```python
from build123d import *

# Parameters (mm, degrees)
F1_DEPTH    = 12.4968
F3_DEPTH    = 152.4
F4_T1_DEPTH = 61.7762374031
F5_R        = 5.08


# Not quite as in the source:
# - a fillet or chamfer that OpenCascade refuses, or shapes differently, is made with other operations: its cross-section is extruded or revolved along the edge and cut away or added
# - a feature names something its author has since deleted; it is built from what else it names


with BuildPart() as f1:
    # F0 (on Top) → F1 (new body)
    with BuildSketch(Plane.XY):
        with BuildLine():
            Line((-93.9849921167, 7.4851757918), (-16.1919427612, 7.4851757918))
            ThreePointArc((-16.1919427612, 7.4851757918), (-15.8959532901, 11.2229099464), (-15.7736930996, 14.9703515835))
            Line((-15.7736930996, 14.9703515835), (-93.9849921167, 14.9703515835))
            Line((-93.9849921167, 14.9703515835), (-93.9849921167, 7.4851757918))
        make_face()
        with BuildLine():
            Line((-93.9849921167, 0), (-17.3162451786, 0))
            ThreePointArc((-17.3162451786, 0), (-16.6663908007, 3.7294145399), (-16.1919427612, 7.4851757918))
            Line((-16.1919427612, 7.4851757918), (-93.9849921167, 7.4851757918))
            Line((-93.9849921167, 7.4851757918), (-93.9849921167, 0))
        make_face()
        Polygon((-93.9849921167, -14.5700745956), (-93.9849921167, 0), (-93.9849921167, 7.4851757918), (-93.9849921167, 14.9703515835), (-93.9849921167, 40.6753872946), (-111.9173921167, 19.2205523892), (-111.9173921167, 14.5700745956), (-111.9173921167, -14.5700745956), align=None)
        with BuildLine():
            Line((-15.7736930996, 14.9703515835), (-8.9203921167, 14.9703515835))
            ThreePointArc((-8.9203921167, 14.9703515835), (-14.3796310702, 36.1097695722), (-23.5038306564, 55.9447705746))
            Line((-23.5038306564, 55.9447705746), (-36.6789735854, 66.7365342379))
            Line((-36.6789735854, 66.7365342379), (-31.7310467362, 54.1373938322))
            ThreePointArc((-31.7310467362, 54.1373938322), (-21.3821676169, 35.5195355237), (-15.7736930996, 14.9703515835))
        make_face()
        with BuildLine():
            Line((-17.3162451786, 0), (-8.9203921167, 0))
            ThreePointArc((-8.9203921167, 0), (-8.270322019, 3.7175238692), (-8.0526666958, 7.4851757917))
            Line((-8.0526666958, 7.4851757918), (-16.1919427612, 7.4851757918))
            ThreePointArc((-16.1919427612, 7.4851757918), (-16.6663908007, 3.7294145399), (-17.3162451786, 0))
        make_face()
        with BuildLine():
            Line((-16.1919427612, 7.4851757918), (-8.0526666958, 7.4851757918))
            ThreePointArc((-8.0526666958, 7.4851757917), (-8.270322019, 11.2528277143), (-8.9203921167, 14.9703515835))
            Line((-8.9203921167, 14.9703515835), (-15.7736930996, 14.9703515835))
            ThreePointArc((-15.7736930996, 14.9703515835), (-15.8959532901, 11.2229099464), (-16.1919427612, 7.4851757918))
        make_face()
        with BuildLine():
            ThreePointArc((-34.6760861576, -35.9113998711), (-16.812117143, -21.5317519133), (-8.9203921167, 0))
            Line((-8.9203921167, 0), (-17.3162451786, 0))
            ThreePointArc((-17.3162451786, 0), (-24.4639001208, -18.231884723), (-37.7452522516, -32.6227247715))
            Line((-37.7452522516, -32.6227247715), (-41.4012260735, -32.6227247715))
            Line((-41.4012260735, -32.6227247715), (-41.4012260735, -41.2478148937))
            Line((-41.4012260735, -41.2478148937), (-39.2100475191, -41.5528100016))
            Line((-39.2100475191, -41.5528100016), (-39.2100475191, -49.5910942554))
            Line((-39.2100475191, -49.5910942554), (-34.6760861576, -49.5910942554))
            Line((-34.6760861576, -49.5910942554), (-34.6760861576, -35.9113998711))
        make_face()
        with BuildLine():
            ThreePointArc((-8.9203921167, 14.9703515835), (-8.270322019, 11.2528277143), (-8.0526666958, 7.4851757917))
            Line((-8.0526666958, 7.4851757918), (16.7025048286, 7.4851757918))
            Line((16.7025048286, 7.4851757918), (16.7025048286, 14.9703515835))
            Line((16.7025048286, 14.9703515835), (-8.9203921167, 14.9703515835))
        make_face()
        with BuildLine():
            ThreePointArc((-8.0526666958, 7.4851757917), (-8.270322019, 3.7175238692), (-8.9203921167, 0))
            Line((-8.9203921167, 0), (16.7025048286, 0))
            Line((16.7025048286, 0), (16.7025048286, 7.4851757918))
            Line((16.7025048286, 7.4851757918), (-8.0526666958, 7.4851757918))
        make_face()
        Polygon((16.7025048286, 7.4851757918), (16.7025048286, 0), (33.5264503956, 7.4851757918), (16.7025048286, 14.9703515835), align=None)
    extrude(amount=F1_DEPTH)

    # F2 (on face) → F3 (cut)
    with BuildSketch(Plane(origin=(-111.9173921167, 0, 0), x_dir=(0, -1, 0), z_dir=(-1, 0, 0))):
        with BuildLine():
            ThreePointArc((-5.9230757918, 6.2484), (-6.3806042889, 7.3529715029), (-7.4851757918, 7.8105))
            Line((-7.4851757918, 7.8105), (-7.4851757918, 4.6863))
            ThreePointArc((-7.4851757918, 4.6863), (-6.3806042889, 5.1438284971), (-5.9230757918, 6.2484))
        make_face()
        with BuildLine():
            Line((-7.4851757918, 4.6863), (-7.4851757918, 7.8105))
            ThreePointArc((-7.4851757918, 7.8105), (-9.0472757918, 6.2484), (-7.4851757918, 4.6863))
        make_face()
    extrude(amount=-F3_DEPTH, mode=Mode.SUBTRACT)

    # F4: fillet of radius 5.08 on 1 edges, made by hand

    # F4_s2 → F4_t1 (cut)
    with BuildSketch(Plane.XY.offset(-28.5449687015)):
        with BuildLine():
            ThreePointArc((23.0943727233, 2.843818927), (26.1093772139, 7.4851757918), (23.0943727233, 12.1265326565))
            Line((23.0943727233, 12.1265326565), (33.5264503956, 7.4851757918))
            Line((33.5264503956, 7.4851757918), (23.0943727233, 2.843818927))
        make_face()
    extrude(amount=F4_T1_DEPTH, mode=Mode.SUBTRACT)

    # F5
    f5_edges = [f1.edges().sort_by_distance(p)[0] for p in [
        (3.891056, 0, 12.4968),
        (3.891056, 14.970352, 12.4968),
        (3.891056, 0, 0),
        (3.891056, 14.970352, 0),
        (-54.879343, 14.970352, 12.4968),
        (-55.650619, 0, 12.4968),
        (-55.650619, 0, 0),
        (-54.879343, 14.970352, 0),
    ]]
    fillet(f5_edges, radius=F5_R)


solid = f1.part
```
Here's how the part is built. I have some questions about the finished solid (model axes, mm). A direction names the side the tool comes from. Round coordinates to 2 decimals unless told otherwise and drop trailing zeros. Order: outer loops, then holes, each group sorted by start corner. A loop starts at its lowest first (then second) coordinate and runs counter-clockwise, first axis right, second up. Notation, with made-up numbers: (7, 17.5) -> (45, 17.5) arc R7 ccw to (45, 28.5) -> close; hole circle Ø6 at (24.25, 32.25). An arc over 180 degrees is marked (long way). Use a Markdown table: item, result. Add a question column.
(1) If we mould it in two halves opening along X, with no side actions, what happens to faces 4 (the face through (-93.985, 28, 6)), 5 (the face through (-59, 9, 0)), 6 (the face through (-23, -15.75, 6.16)), 7 (the face through (-29.999, 61.265, 6.161))? For each: released by +X, released by -X, zero draft, split by the parting line, or undercut.
(2) Suppose I cut it at D-D, the plane z = 10.25. Please give me the cut outline in (x, y) (3 decimals), and give its area (3 significant figures).
(3) Suppose I cut it at B-B, the plane x = -25.5. Please give me the cut outline in (y, z), and give its area (3 significant figures).
(4) For faces 1 (the face through (-55.132, 13.522, 1.528)), 2 (the face through (4.23, 13.44, 11.05)), 3 (the face through (4.226, 13.443, 1.449)), which set-ups out of +Z, -Z, +X, -X, +Y, -Y let a thin tool reach every point of the face, with its end or its side?
(5) Suppose I cut it at A-A, the plane x = -5. Please give me the cut outline in (y, z), and give its area (3 significant figures).
(6) For pin 1 Ø7 at (y, z) = (-36, 5) entering from -X; pin 2 Ø1.5 at (x, z) = (-33.5, 2) entering from +Y; pin 3 Ø4 at (x, y) = (-81.5, -0.5) entering from +Z; pin 4 Ø2 at (y, z) = (-15, 8.5) entering from -X, each with a flat end and sliding along its axis, tell me the tip position at first contact or that it passes through.
(7) Suppose I cut it at C-C, the plane y = -3.5. Please give me the cut outline in (x, z) (3 decimals), and give its area (3 significant figures).
(8) I need wall thicknesses on line 1 along Y through (x, z) = (-22, 7); line 2 along X through (y, z) = (-41, 3.5); line 3 along Y through (x, z) = (1, 7.5). Which ranges of each line are inside material? Lowest first, please.
Verdict:
| question | item | result |
|---|---|---|
| 1 | face 4 | undercut |
| 1 | face 5 | zero draft |
| 1 | face 6 | undercut |
| 1 | face 7 | released by +X |
| 2 | outline | (-111.917, -14.57) -> (-93.985, -14.57) -> (-93.985, 0.863) -> (-17.16, 0.863) arc R52.989 cw to (-37.745, -32.623) -> (-41.401, -32.623) -> (-41.401, -41.248) -> (-39.21, -41.553) -> (-39.21, -49.591) -> (-34.676, -49.591) -> (-34.676, -35.911) arc R42.854 ccw to (-8.86, 0.863) -> (18.643, 0.863) -> (23.094, 2.844) arc R5.08 ccw to (23.094, 12.127) -> (18.643, 14.107) -> (-8.781, 14.107) arc R122.534 ccw to (-23.504, 55.945) -> (-36.679, 66.737) -> (-31.731, 54.137) arc R88.64 cw to (-15.651, 14.107) -> (-93.985, 14.107) -> (-93.985, 40.675) -> (-111.917, 19.221) -> close |
| 2 | area | 3,150 mm2 |
| 3 | outline | (-30.52, 0) -> (-19.82, 0) -> (-19.82, 12.5) -> (-30.52, 12.5) -> close; (0, 5.08) arc R5.08 ccw to (5.08, 0) -> (9.89, 0) arc R5.08 ccw to (14.97, 5.08) -> (14.97, 7.42) arc R5.08 ccw to (9.89, 12.5) -> (5.08, 12.5) arc R5.08 ccw to (0, 7.42) -> close; (44.24, 0) -> (57.58, 0) -> (57.58, 12.5) -> (44.24, 12.5) -> close; hole circle Ø3.12 at (7.49, 6.25) |
| 3 | area | 458 mm2 |
| 4 | face 1 | -Z |
| 4 | face 2 | +Z, +X, +Y |
| 4 | face 3 | -Z, +X, +Y |
| 5 | outline | (0, 5.08) arc R5.08 ccw to (5.08, 0) -> (9.89, 0) arc R5.08 ccw to (14.97, 5.08) -> (14.97, 7.42) arc R5.08 ccw to (9.89, 12.5) -> (5.08, 12.5) arc R5.08 ccw to (0, 7.42) -> close; hole circle Ø3.12 at (7.49, 6.25) |
| 5 | area | 157 mm2 |
| 6 | pin 1 | x = -41.4 |
| 6 | pin 2 | y = 64.75 |
| 6 | pin 3 | z = 11.02 |
| 6 | pin 4 | x = -111.92 |
| 7 | outline | (-111.917, 0) -> (-93.985, 0) -> (-93.985, 12.497) -> (-111.917, 12.497) -> close; (-18.105, 0) -> (-9.348, 0) -> (-9.348, 12.497) -> (-18.105, 12.497) -> close |
| 7 | area | 334 mm2 |
| 8 | line 1 | -27.51 to -13.85, 0 to 6.12, 8.85 to 14.97, 37 to 53.24 |
| 8 | line 2 | -41.4 to -34.68 |
| 8 | line 3 | 0 to 6.55, 8.42 to 14.97 |
